Build history of the part. All positions in model axes, mm. A direction names the side the tool comes from. Give positions to 0.01 mm unless a question says otherwise; leave off trailing zeros. Write each loop counter-clockwise with the first axis right and the second up, starting at its lowest first coordinate (ties: lowest second). Pieces come first, ordered by that corner, then holes. Notation, with made-up numbers: (-35.75, 65) -> (0.25, 65) arc R26 ccw to (0.25, 86) -> close; hole circle Ø10 at (55.5, -29.5). An arc over 180 degrees is marked (long way). Write item = value, one per line. Start each with the question number.
Q1. Drop flat-ended pins along their axis: P1, Ø0.9, axis at x = 29.5, z = -7.5, coming from the +Y side; P2, Ø2.5, axis at x = 30, z = -1.5, coming from the +Y side; P3, Ø1.5, axis at x = 31, y = 2, coming from the -Z side. Give the stop position or say it passes through.
Q2. Saw through at C-C, the plane z = -6.75. List the corners of the cut face in (x, y), then the cut area to 3 significant figures.
Q3. Saw through at B-B, the plane x = 28.5. List the corners of the cut face in (y, z), then the cut area to 3 significant figures.
Q4. Wall check: line 1 (Z direction, x = 28.5, y = 3.9); line 2 (Y direction, x = 28.75, z = -1.75); line 3 (Z direction, x = 27, y = 1.45). Give the ranges that are in metal, low to high.
Q5. Tool access for faces 1 (the face through (26.84, 3.03, -2.8)), 2 (the face through (33.268, 3.028, -6.199)), 3 (the face through (30, 3, -2.5)): list every direction of +Z, -Z, +X, -X, +Y, -Y with a clear straight run to the whole face (end or side of a thin tool).
Q6. Saw through at A-A, the plane y = 2.1. List the corners of the cut face in (x, z).
Q7. Saw through at D-D, the plane z = -0.75. List the corners of the cut face in (x, y).
from build123d import *

# Parameters (mm, degrees)
SKETCH_1_W          = 7
SKETCH_1_H          = 8
EXTRUDE_1_DEPTH     = 1
EXTRUDE_2_DEPTH     = 4.5
FILLET_1_R          = 1
FILLET_2_R          = 0.5
CUT_EXTRUDE_START   = -0.5
CUT_EXTRUDE_1_DEPTH = 0.5


with BuildPart() as part:
    # 草图1 → 凸台-拉伸1 (new body)
    with BuildSketch(Plane(origin=(0, 0, 0), x_dir=(1, 0, 0), z_dir=(0, 1, 0))):
        with Locations((30.052937772, 4.5)):
            Rectangle(SKETCH_1_W, SKETCH_1_H)
    extrude(amount=EXTRUDE_1_DEPTH)

    # 草图2 → 凸台-拉伸2 (add)
    with BuildSketch(Plane(origin=(0, 1, 0), x_dir=(1, 0, 0), z_dir=(0, 1, 0))):
        Polygon((26.552937772, 4.5), (26.552937772, 6.5), (33.552937772, 6.5), (33.552937772, 2.5), (26.552937772, 2.5), align=None)
    extrude(amount=EXTRUDE_2_DEPTH)

    # 圆角1
    fillet_1_edges = [part.edges().sort_by_distance(p)[0] for p in [
        (26.552937772, 3.25, -2.5),
        (33.552937772, 3.25, -2.5),
        (33.552937772, 3.25, -6.5),
        (26.552937772, 3.25, -6.5),
        (26.552937772, 0.5, -8.5),
        (33.552937772, 0.5, -8.5),
        (33.552937772, 0.5, -0.5),
        (26.552937772, 0.5, -0.5),
    ]]
    fillet(fillet_1_edges, radius=FILLET_1_R)

    # 圆角2
    fillet_2_edges = [part.edges().sort_by_distance(p)[0] for p in [
        (26.552937772, 5.5, -4.5),
        (30.052937772, 5.5, -6.5),
        (30.052937772, 5.5, -2.5),
        (33.552937772, 5.5, -4.5),
        (33.260044553, 5.5, -6.207106781),
        (33.260044553, 5.5, -2.792893219),
        (26.84583099, 5.5, -2.792893219),
        (26.84583099, 5.5, -6.207106781),
    ]]
    fillet(fillet_2_edges, radius=FILLET_2_R)

    # 草图3 → 切除-拉伸1 (cut)
    with BuildSketch(Plane.XZ.offset(CUT_EXTRUDE_START)):
        with BuildLine():
            Line((26.552937772, -1.5), (26.552937772, -7.5))
            ThreePointArc((26.552937772, -7.5), (26.84583099, -8.207106781), (27.552937772, -8.5))
            Line((27.552937772, -8.5), (32.552937772, -8.5))
            ThreePointArc((32.552937772, -8.5), (33.260044553, -8.207106781), (33.552937772, -7.5))
            Line((33.552937772, -7.5), (33.552937772, -1.5))
            ThreePointArc((33.552937772, -1.5), (33.260044553, -0.792893219), (32.552937772, -0.5))
            Line((32.552937772, -0.5), (27.552937772, -0.5))
            ThreePointArc((27.552937772, -0.5), (26.84583099, -0.792893219), (26.552937772, -1.5))
        make_face()
    extrude(amount=CUT_EXTRUDE_1_DEPTH, mode=Mode.SUBTRACT)


solid = part.part
Report:
q1.P1 = 1
q1.P2 = 5.43
q1.P3 = -6.5
q2.outline = (26.55, 0.5) -> (33.55, 0.5) -> (33.55, 1) -> (26.55, 1) -> close
q2.area = 3.50 mm2
q3.outline = (0.5, -8.5) -> (1, -8.5) -> (1, -6.5) -> (5, -6.5) arc R0.5 ccw to (5.5, -6) -> (5.5, -3) arc R0.5 ccw to (5, -2.5) -> (1, -2.5) -> (1, -0.5) -> (0.5, -0.5) -> close
q3.area = 21.9 mm2
q4.line_1 = -6.5 to -2.5
q4.line_2 = 0.5 to 1
q4.line_3 = -6.33 to -2.67
q5.face_1 = +Z, -X, +Y
q5.face_2 = -Z, +X, +Y
q5.face_3 = +Z, +X, -X, +Y
q6.outline = (26.55, -5.5) arc R1 ccw to (27.55, -6.5) -> (32.55, -6.5) arc R1 ccw to (33.55, -5.5) -> (33.55, -3.5) arc R1 ccw to (32.55, -2.5) -> (27.55, -2.5) arc R1 ccw to (26.55, -3.5) -> close
q7.outline = (26.89, 0.5) -> (33.21, 0.5) -> (33.21, 1) -> (26.89, 1) -> close
